The drawing under review shows one solid part. Ordinate dimensions are in mm from its lowest x, y, z. Coordinates: 2 decimals unless noted, no trailing zeros. Loops run counter-clockwise (first coordinate to the right, second up) from the corner with the lowest first, then second, coordinate; pieces in that order, holes last. Notation, with made-up numbers: M -20,78.25 L 2,78.25 A19 cw 2,98.25 Z; hole C 33,84.25 d10. An arc over 180 degrees is marked long. Answer as a JSON object with one key per item and string values. Group by question number.
1. Consider section A-A (y = 56). State the section outline as (x, z) points.
2. Consider section C-C (x = 36). State the section outline as (y, z) points, then the cut area to 3 significant figures.
3. Consider section B-B (x = 20.5). State the section outline as (y, z) points, then the cut area to 3 significant figures.
4. To check wall thickness, follow probe 1 along X at (y, z) = (48.5, 2.25); probe 2 along Y at (x, z) = (36, 1.65); probe 3 along Y at (x, z) = (28, 0.6). State the ranges of each line that lie inside material, in increasing order.
5. Consider section D-D (z = 1.8). State the section outline as (x, y) points.
6. Insertion check: pin 1 (1 mm diameter, centred on y = 52.5, z = 0.5, fed in from -X). The pin has a flat end and moves straight along its axis. Give the tip position at first contact, or say it passes through.
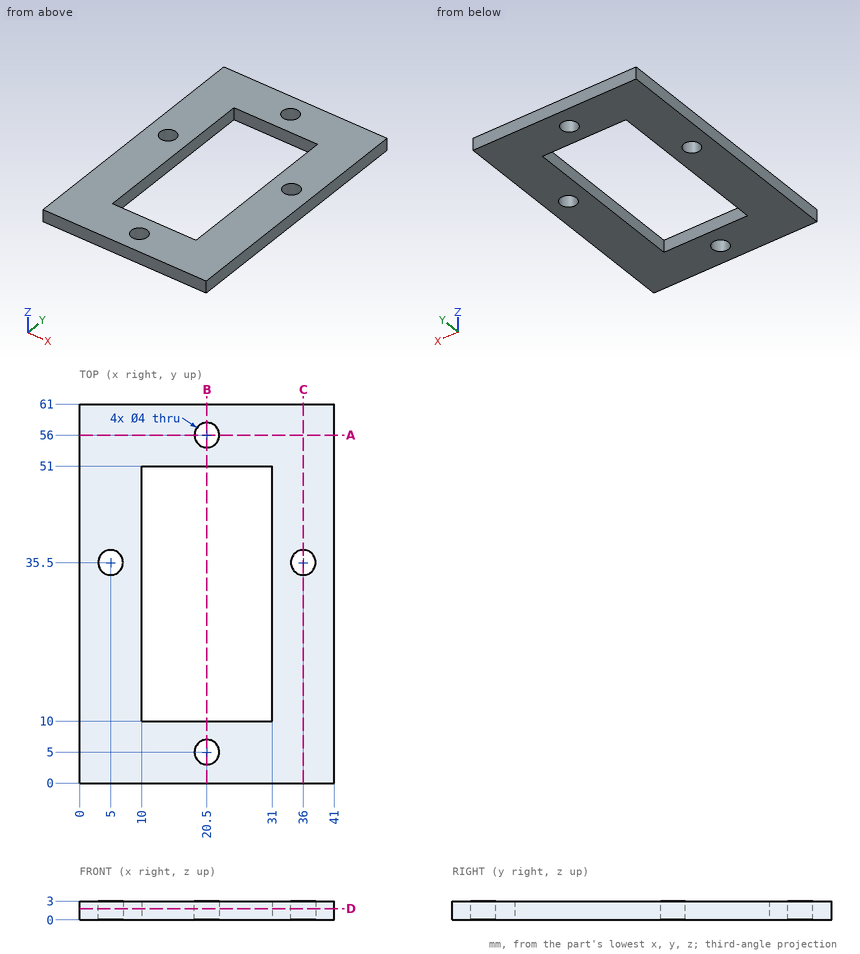
Findings below:
{
 "1": {"outline": "M 0,0 L 18.5,0 L 18.5,3 L 0,3 Z; M 22.5,0 L 41,0 L 41,3 L 22.5,3 Z"},
 "2": {"outline": "M 0,0 L 33.5,0 L 33.5,3 L 0,3 Z; M 37.5,0 L 61,0 L 61,3 L 37.5,3 Z", "area": "171 mm^2"},
 "3": {"outline": "M 0,0 L 3,0 L 3,3 L 0,3 Z; M 7,0 L 10,0 L 10,3 L 7,3 Z; M 51,0 L 54,0 L 54,3 L 51,3 Z; M 58,0 L 61,0 L 61,3 L 58,3 Z", "area": "36.0 mm^2"},
 "4": {"probe 1": "x = 0 to 10, 31 to 41", "probe 2": "y = 0 to 33.5, 37.5 to 61", "probe 3": "y = 0 to 10, 51 to 61"},
 "5": {"outline": "M 0,0 L 41,0 L 41,61 L 0,61 Z; hole C 5,35.5 d4; hole M 10,10 L 31,10 L 31,51 L 10,51 Z; hole C 20.5,5 d4; hole C 20.5,56 d4; hole C 36,35.5 d4"},
 "6": {"pin 1": "stops at x = 0"}
}
